from build123d import *

# Parameters (mm, degrees)
SKETCH1_W           = 4.5
SKETCH1_H           = 3
BOSS_EXTRUDE1_DEPTH = 3


with BuildPart() as part:
    # Sketch1 → Boss-Extrude1 (new body)
    with BuildSketch(Plane.XY):
        with BuildLine():
            Line((18, 157.5), (15, 157.5))
            Line((15, 157.5), (15, 154.5))
            Line((15, 154.5), (18, 154.5))
            Line((18, 154.5), (18, 145.5))
            Line((18, 145.5), (15, 145.5))
            Line((15, 145.5), (15, 142.5))
            Line((15, 142.5), (18, 142.5))
            Line((18, 142.5), (18, 133.5))
            Line((18, 133.5), (15, 133.5))
            Line((15, 133.5), (15, 130.5))
            Line((15, 130.5), (18, 130.5))
            Line((18, 130.5), (18, 121.5))
            Line((18, 121.5), (15, 121.5))
            Line((15, 121.5), (15, 118.5))
            Line((15, 118.5), (18, 118.5))
            Line((18, 118.5), (18, 109.5))
            Line((18, 109.5), (15, 109.5))
            Line((15, 109.5), (15, 106.5))
            Line((15, 106.5), (18, 106.5))
            Line((18, 106.5), (18, 97.5))
            Line((18, 97.5), (15, 97.5))
            Line((15, 97.5), (15, 94.5))
            Line((15, 94.5), (18, 94.5))
            Line((18, 94.5), (18, 85.5))
            Line((18, 85.5), (15, 85.5))
            Line((15, 85.5), (15, 82.5))
            Line((15, 82.5), (18, 82.5))
            Line((18, 82.5), (18, 73.5))
            Line((18, 73.5), (15, 73.5))
            Line((15, 73.5), (15, 70.5))
            Line((15, 70.5), (18, 70.5))
            Line((18, 70.5), (18, 67.5))
            Line((18, 67.5), (10.5, 67.5))
            Line((10.5, 67.5), (10.5, 64.5))
            Line((10.5, 64.5), (18, 64.5))
            Line((18, 64.5), (18, 61.5))
            Line((18, 61.5), (15, 58.5))
            ThreePointArc((15, 58.5), (9.968847051, 57.312305899), (6, 54))
            Line((6, 54), (6, 70.5))
            Line((6, 70.5), (3, 70.5))
            Line((3, 70.5), (3, 73.5))
            Line((3, 73.5), (6, 73.5))
            Line((6, 73.5), (6, 106.5))
            Line((6, 106.5), (3, 106.5))
            Line((3, 106.5), (3, 109.5))
            Line((3, 109.5), (6, 109.5))
            Line((6, 109.5), (6, 130.5))
            Line((6, 130.5), (3, 130.5))
            Line((3, 130.5), (3, 133.5))
            Line((3, 133.5), (6, 133.5))
            Line((6, 133.5), (6, 166.5))
            Line((6, 166.5), (3, 166.5))
            Line((3, 166.5), (3, 169.5))
            Line((3, 169.5), (6, 169.5))
            Line((6, 169.5), (6, 172.5))
            Line((6, 172.5), (10.5, 172.5))
            Line((10.5, 172.5), (10.5, 175.5))
            Line((10.5, 175.5), (6, 175.5))
            Line((6, 175.5), (6, 186))
            ThreePointArc((6, 186), (9.968847051, 182.687694101), (15, 181.5))
            Line((15, 181.5), (18, 178.5))
            Line((18, 178.5), (18, 169.5))
            Line((18, 169.5), (15, 169.5))
            Line((15, 169.5), (15, 166.5))
            Line((15, 166.5), (18, 166.5))
            Line((18, 166.5), (18, 157.5))
        make_face()
        with Locations((12.75, 78)):
            Rectangle(SKETCH1_W, SKETCH1_H, mode=Mode.SUBTRACT)
        with Locations((12.75, 162)):
            Rectangle(SKETCH1_W, SKETCH1_H, mode=Mode.SUBTRACT)
        with Locations((12.75, 150)):
            Rectangle(SKETCH1_W, SKETCH1_H, mode=Mode.SUBTRACT)
        with Locations((12.75, 138)):
            Rectangle(SKETCH1_W, SKETCH1_H, mode=Mode.SUBTRACT)
        with Locations((12.75, 126)):
            Rectangle(SKETCH1_W, SKETCH1_H, mode=Mode.SUBTRACT)
        with Locations((12.75, 114)):
            Rectangle(SKETCH1_W, SKETCH1_H, mode=Mode.SUBTRACT)
        with Locations((12.75, 102)):
            Rectangle(SKETCH1_W, SKETCH1_H, mode=Mode.SUBTRACT)
        with Locations((12.75, 90)):
            Rectangle(SKETCH1_W, SKETCH1_H, mode=Mode.SUBTRACT)
    extrude(amount=BOSS_EXTRUDE1_DEPTH)


solid = part.part
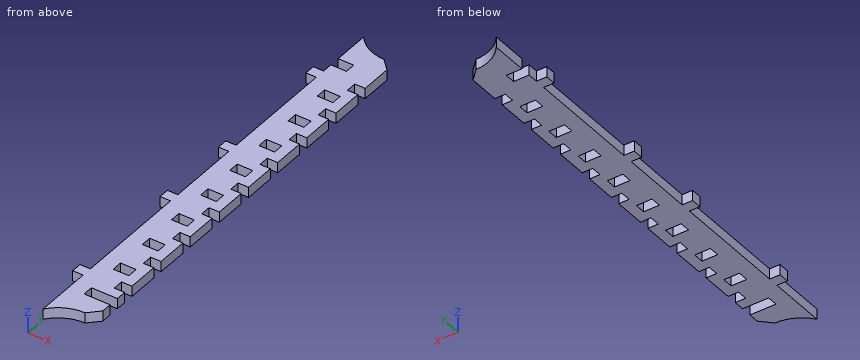
Source: CAD feature listing. Evaluate the final solid. Frame: model axes, mm. Coordinates: 2 decimals unless noted, no trailing zeros. Loops run counter-clockwise (first coordinate to the right, second up) from the corner with the lowest first, then second, coordinate; pieces in that order, holes last. Notation, with made-up numbers: (47, 52.5) - (100, 52.5) arc R7 cw to (100, 64.5) - close; hole circle Ø2 at (68.5, -17). An arc over 180 degrees is marked (long way). Return JSON: item names as keys, results as strings.
Q1. Section A-A, the plane y = 102. Return loops of the section in (x, z).
Results:
{"outline": "(6, 0) - (10.5, 0) - (10.5, 3) - (6, 3) - close; (15, 0) - (18, 0) - (18, 3) - (15, 3) - close"}
Q2. Material intervals for line 1 along Y through (x, z) = (4.5, 0.4); line 2 along X through (y, z) = (163, 0.9); line 3 along X through (y, z) = (63, 1.75), sorted ascending.
Results:
{"line 1": "70.5 to 73.5, 106.5 to 109.5, 130.5 to 133.5, 166.5 to 169.5", "line 2": "6 to 10.5, 15 to 18", "line 3": "6 to 18"}
Q3. Section B-B, the plane x = 7.25. Return loops of the section in (y, z), plus the area to 3 significant figures.
Results:
{"outline": "(55.4, 0) - (172.5, 0) - (172.5, 3) - (55.4, 3) - close; (175.5, 0) - (184.6, 0) - (184.6, 3) - (175.5, 3) - close", "area": "379 mm2"}
Q4. Section C-C, the plane x = 16.5. Give the number of separate pieces and of enclosed holes in the cut face, plus the area to 3 significant figures.
Results:
{"separate pieces": "11", "enclosed holes": "0", "area": "270 mm2"}
Q5. Contact query for flat-ended pins moving along their axis: P1, Ø1.5, axis at y = 155, z = 1, coming from the +X side; P2, Ø1.5, axis at x = 13.5, z = 1.5, coming from the +Y side; P3, Ø1.5, axis at y = 167.5, z = 1, coming from the +X side; P4, Ø0.9, axis at y = 125.5, z = 1, coming from the -X side. Output: stop coordinate, or through.
Results:
{"P1": "x = 18", "P2": "y = 181.73", "P3": "x = 15", "P4": "x = 6"}
